```python
from build123d import *

# Parameters (mm, degrees)
BOSS_EXTRUDE1_DEPTH = 1
SKETCH2_W           = 1.5
SKETCH2_H           = 0.3
CUT_EXTRUDE1_DEPTH  = 1


with BuildPart() as part:
    # Sketch1 → Boss-Extrude1 (new body)
    with BuildSketch(Plane(origin=(0, 0, 0), x_dir=(1, 0, 0), z_dir=(0, 1, 0))):
        with BuildLine():
            Line((0, 1), (10, 1))
            ThreePointArc((10, 1), (10.499999999, 1.499999999), (10, 1.999999998))
            ThreePointArc((10, 1.999999998), (8.5, 3.499999998), (10, 4.999999998))
            add(Edge.make_bspline(
                [(10, 4.999999998), (14.475567746, 4.998166583), (17.999999995, 1)],
                knots=[0, 0, 0, 1, 1, 1], degree=2))
            Line((17.999999995, 1), (24, 1))
            ThreePointArc((24, 1), (24.499999999, 1.5), (24, 1.999999999))
            ThreePointArc((24, 1.999999999), (22.500000001, 3.500000002), (24.000000003, 5))
            add(Edge.make_bspline(
                [(24.000000003, 5), (28.47556775, 4.998166585), (31.999999998, 1)],
                knots=[0, 0, 0, 1, 1, 1], degree=2))
            Line((31.999999998, 1), (41.999999998, 1))
            Line((41.999999998, 1), (41.999999998, -1.000000004))
            Line((41.999999998, -1.000000004), (31.999999996, -1.000000004))
            add(Edge.make_bspline(
                [(23.999999999, -5), (28.475567744, -4.998166004), (31.999999996, -1.000000004)],
                knots=[0, 0, 0, 1, 1, 1], degree=2))
            ThreePointArc((23.999999999, -5), (22.499999999, -3.5), (23.999999999, -2))
            ThreePointArc((23.999999999, -2), (24.499999999, -1.5), (23.999999999, -1))
            Line((23.999999999, -1), (17.999999995, -1))
            add(Edge.make_bspline(
                [(10, -4.999999998), (14.475567746, -4.998166584), (17.999999995, -1)],
                knots=[0, 0, 0, 1, 1, 1], degree=2))
            ThreePointArc((10, -4.999999998), (8.50000001, -3.500000008), (10, -2.000000018))
            ThreePointArc((10, -2.000000018), (10.500000009, -1.500000009), (10, -1))
            Line((10, -1), (0, -1))
            Line((0, -1), (0, -0.1))
            Line((0, -0.1), (4, -0.1))
            Line((4, -0.1), (4, 0.1))
            Line((4, 0.1), (0, 0.1))
            Line((0, 0.1), (0, 1))
        make_face()
    extrude(amount=BOSS_EXTRUDE1_DEPTH)

    # Sketch2 → Cut-Extrude1 (cut)
    with BuildSketch(Plane(origin=(0, 1, 0), x_dir=(1, 0, 0), z_dir=(0, 1, 0))):
        with Locations((15.932882113, 0.071093436)):
            Rectangle(SKETCH2_W, SKETCH2_H)
        with Locations((30.000000004, 3e-09)):
            Rectangle(SKETCH2_W, SKETCH2_H)
        with BuildLine():
            ThreePointArc((10, -3.699999998), (13.699999998, 0), (10, 3.699999998))
            ThreePointArc((10, 3.699999998), (9.800000001, 3.499999999), (10, 3.3))
            ThreePointArc((10, 3.3), (13.3, 0), (10, -3.3))
            ThreePointArc((10, -3.3), (9.800000001, -3.499999999), (10, -3.699999998))
        make_face()
        with BuildLine():
            ThreePointArc((24, -3.699999998), (27.699999998, 0), (24, 3.699999998))
            ThreePointArc((24, 3.699999998), (23.8, 3.499999998), (24, 3.299999998))
            ThreePointArc((24, 3.299999998), (27.299999998, 0), (24, -3.299999998))
            ThreePointArc((24, -3.299999998), (23.8, -3.499999998), (24, -3.699999998))
        make_face()
    extrude(amount=-CUT_EXTRUDE1_DEPTH, mode=Mode.SUBTRACT)


solid = part.part
```
CAD build for the part. Positions are in the model's coordinates, mm. A direction names the side the tool comes from. Give positions to 0.01 mm unless a question says otherwise; leave off trailing zeros. Loops run counter-clockwise (first coordinate to the right, second up) from the corner with the lowest first, then second, coordinate; pieces in that order, holes last. Notation, with made-up numbers: (21, 57) -> (39, 57) arc R21 ccw to (39, 62) -> close; hole circle Ø3 at (27, -32). An arc over 180 degrees is marked (long way). Use a Markdown table: item, result.
1. Slice it at A-A (x = 3.5). List the corners of the cut face in (y, z).
Check result:
| item | result |
|---|---|
| outline | (0, -1) -> (1, -1) -> (1, -0.1) -> (0, -0.1) -> close; (0, 0.1) -> (1, 0.1) -> (1, 1) -> (0, 1) -> close |
2. Mould opens along Z. For faces 1 (the flat face through (42, 0.5, 0)), 2 (the flat face through (37.1, 0.5, 1)), 3 (the flat face through (36.9, 0.5, -1)), 4 (the cylindrical face through (13.7, 0.5, 0.1)) say: pulls with the +Z half, pulls with the -Z half, needs draft (parallel to the pull), parting line crosses it, or undercut.
Check result:
| item | result |
|---|---|
| face 1 | needs draft |
| face 2 | pulls with the +Z half |
| face 3 | pulls with the -Z half |
| face 4 | undercut |
3. Which spindle directions (+Z, -Z, +X, -X, +Y, -Y) get a long thin tool onto all of the face, cutting with end or side? Do faces 5 (the flat face through (2, 0.5, -0.1)), 6 (the flat face through (21, 0.5, 1)), 7 (the flat face through (0, 0.5, 0.6)). Say none if no direction does.
Check result:
| item | result |
|---|---|
| face 5 | -X, +Y, -Y |
| face 6 | +Y, -Y |
| face 7 | +Z, -Z, -X, +Y, -Y |
4. Flat gauge pins, fed straight in: pin 1 (1 mm diameter, centred on x = 34, z = -3, fed in from +Y); pin 2 (0.5 mm diameter, centred on x = 21.5, y = 0.5, fed in from -Z); pin 3 (0.5 mm diameter, centred on x = 2.5, y = 0.5, fed in from +Z). Where does each tip first touch, or does it go through?
Check result:
| item | result |
|---|---|
| pin 1 | passes through |
| pin 2 | stops at z = -1 |
| pin 3 | stops at z = 1 |
5. Wall check: L1, parallel to X at y = 0.35, z = -2.5; L2, parallel to Z at x = 3.5, y = 0.9; L3, parallel to Z at x = 13, y = 0.4. Give the ranges that are in metal, low to high. Write a range as [from, to].
Check result:
| item | result |
|---|---|
| L1 | x = [8.88, 12.15], [12.73, 16.48], [22.88, 26.15], [26.73, 30.48] |
| L2 | z = [-1, -0.1], [0.1, 1] |
| L3 | z = [-4.51, -2.17], [-1.37, 1.37], [2.17, 4.51] |
6. Slice it at B-B (y = 0.3). Give the number of separate pieces and of enclosed holes in the cut face, plus the area to 3 significant figures.
Check result:
| item | result |
|---|---|
| separate pieces | 1 |
| enclosed holes | 4 |
| area | 174 mm^2 |
